```python
from build123d import *

# Parameters (mm, degrees)
SKETCH2_R           = 11.1125
BOSS_EXTRUDE1_DEPTH = 6.35


with BuildPart() as part:
    # Sketch2 → Boss-Extrude1 (new body)
    with BuildSketch(Plane.XY):
        with BuildLine():
            Line((0, 914.4), (-194.479849892, 914.4))
            ThreePointArc((-194.479849892, 914.4), (-204.91887294, 907.625287079), (-202.983200568, 895.332073104))
            ThreePointArc((-202.983200568, 895.332073104), (-164.535916973, 779.903104595), (-165.892020397, 658.247026365))
            Line((-165.892020397, 658.247026365), (-165.938886188, 658.129795086))
            ThreePointArc((-165.938886188, 658.129795086), (-174.522720833, 620.054602536), (-187.919807247, 583.395080165))
            ThreePointArc((-187.919807247, 583.395080165), (-210.62430537, 541.201744159), (-239.683438479, 503.105305725))
            ThreePointArc((-239.683438479, 503.105305725), (-421.799875663, 296.628923536), (-582.037423098, 72.747657042))
            ThreePointArc((-582.037423098, 72.747657042), (-620.339092238, 32.211350912), (-671.307126152, 9.573561873))
            ThreePointArc((-671.307126152, 9.573561873), (-674.990888604, 5.409489794), (-676.274252252, 0))
            ThreePointArc((-676.274252252, 0), (-674.990888604, -5.409489794), (-671.307126152, -9.573561873))
            ThreePointArc((-671.307126152, -9.573561873), (-620.339092238, -32.211350912), (-582.037423098, -72.747657042))
            ThreePointArc((-582.037423098, -72.747657042), (-421.799875663, -296.628923536), (-239.683438479, -503.105305725))
            ThreePointArc((-239.683438479, -503.105305725), (-191.627212465, -575.297388544), (-165.938886188, -658.129795086))
            Line((-165.938886188, -658.129795086), (-165.892020397, -658.247026365))
            ThreePointArc((-165.892020397, -658.247026365), (-164.535916973, -779.903104595), (-202.983200568, -895.332073104))
            ThreePointArc((-202.983200568, -895.332073104), (-204.91887294, -907.625287079), (-194.479849892, -914.4))
            Line((-194.479849892, -914.4), (0, -914.4))
            Line((0, -914.4), (194.479849892, -914.4))
            ThreePointArc((194.479849892, -914.4), (204.91887294, -907.625287079), (202.983200568, -895.332073104))
            ThreePointArc((202.983200568, -895.332073104), (164.535916973, -779.903104595), (165.892020397, -658.247026365))
            Line((165.892020397, -658.247026365), (165.938886188, -658.129795086))
            ThreePointArc((165.938886188, -658.129795086), (174.522720833, -620.054602536), (187.919807247, -583.395080165))
            ThreePointArc((187.919807247, -583.395080165), (210.62430537, -541.201744159), (239.683438479, -503.105305725))
            ThreePointArc((239.683438479, -503.105305725), (421.799875663, -296.628923536), (582.037423098, -72.747657043))
            ThreePointArc((582.037423098, -72.747657043), (620.339092238, -32.211350912), (671.307126152, -9.573561873))
            ThreePointArc((671.307126152, -9.573561873), (674.990888603, -5.409489794), (676.274252252, 0))
            ThreePointArc((676.274252252, 0), (674.990888604, 5.409489794), (671.307126152, 9.573561873))
            ThreePointArc((671.307126152, 9.573561873), (620.339092238, 32.211350912), (582.037423098, 72.747657042))
            ThreePointArc((582.037423098, 72.747657042), (421.799875663, 296.628923536), (239.683438479, 503.105305725))
            ThreePointArc((239.683438479, 503.105305725), (191.627212465, 575.297388544), (165.938886188, 658.129795086))
            Line((165.938886188, 658.129795086), (165.892020397, 658.247026365))
            ThreePointArc((165.892020397, 658.247026365), (164.535916973, 779.903104595), (202.983200568, 895.332073104))
            ThreePointArc((202.983200568, 895.332073104), (204.91887294, 907.625287079), (194.479849892, 914.4))
            Line((194.479849892, 914.4), (0, 914.4))
        make_face()
        with Locations((-58.541769794, -639.405335996)):
            Circle(SKETCH2_R, mode=Mode.SUBTRACT)
        with Locations((-58.541769794, -838.268909678)):
            Circle(SKETCH2_R, mode=Mode.SUBTRACT)
        with Locations((58.541769794, -838.268909678)):
            Circle(SKETCH2_R, mode=Mode.SUBTRACT)
        with Locations((58.541769794, -639.405335996)):
            Circle(SKETCH2_R, mode=Mode.SUBTRACT)
        with Locations((533.590599666, -57.767812484)):
            Circle(SKETCH2_R, mode=Mode.SUBTRACT)
        with Locations((330.356144827, -56.532187516)):
            Circle(SKETCH2_R, mode=Mode.SUBTRACT)
        with Locations((330.356144827, 56.532187516)):
            Circle(SKETCH2_R, mode=Mode.SUBTRACT)
        with Locations((533.590599666, 57.767812484)):
            Circle(SKETCH2_R, mode=Mode.SUBTRACT)
        with Locations((58.541769794, 838.268909678)):
            Circle(SKETCH2_R, mode=Mode.SUBTRACT)
        with Locations((-58.541769794, 838.268909678)):
            Circle(SKETCH2_R, mode=Mode.SUBTRACT)
        with Locations((-58.541769794, 639.405335996)):
            Circle(SKETCH2_R, mode=Mode.SUBTRACT)
        with Locations((58.541769794, 639.405335996)):
            Circle(SKETCH2_R, mode=Mode.SUBTRACT)
        with Locations((-330.356144827, -56.532187516)):
            Circle(SKETCH2_R, mode=Mode.SUBTRACT)
        with Locations((-330.356144827, 56.532187516)):
            Circle(SKETCH2_R, mode=Mode.SUBTRACT)
        with Locations((-533.590599666, 57.767812484)):
            Circle(SKETCH2_R, mode=Mode.SUBTRACT)
        with Locations((-533.590599666, -57.767812484)):
            Circle(SKETCH2_R, mode=Mode.SUBTRACT)
        with BuildLine():
            Line((294.116579618, 52.07611641), (294.116579618, -52.07611641))
            ThreePointArc((294.116579618, -52.07611641), (242.916605185, -291.544447454), (101.6983636, -491.604256507))
            ThreePointArc((101.6983636, -491.604256507), (89.07407881, -503.133976698), (76.131755899, -514.305516063))
            ThreePointArc((76.131755899, -514.305516063), (40.620898237, -536.014461284), (0, -545.083195538))
            ThreePointArc((0, -545.083195538), (-40.620898237, -536.014461284), (-76.131755899, -514.305516063))
            ThreePointArc((-76.131755899, -514.305516063), (-235.841357727, -307.108762007), (-294.116579618, -52.07611641))
            Line((-294.116579618, -52.07611641), (-294.116579618, 52.07611641))
            ThreePointArc((-294.116579618, 52.07611641), (-242.916605185, 291.544447454), (-101.6983636, 491.604256507))
            ThreePointArc((-101.6983636, 491.604256507), (-89.07407881, 503.133976698), (-76.131755899, 514.305516063))
            ThreePointArc((-76.131755899, 514.305516063), (-40.620898237, 536.014461284), (0, 545.083195538))
            ThreePointArc((0, 545.083195538), (40.620898237, 536.014461284), (76.131755899, 514.305516063))
            ThreePointArc((76.131755899, 514.305516063), (235.841357727, 307.108762007), (294.116579618, 52.07611641))
        make_face(mode=Mode.SUBTRACT)
    extrude(amount=BOSS_EXTRUDE1_DEPTH)


solid = part.part
```
The model under review builds one solid part; all positions refer to its coordinate system, in mm. A direction names the side the tool comes from. Give positions to 0.01 mm unless a question says otherwise; leave off trailing zeros. Write each loop counter-clockwise with the first axis right and the second up, starting at its lowest first coordinate (ties: lowest second). Pieces come first, ordered by that corner, then holes.
(1) Consider section D-D, the plane x = 461. Give the boundary of the cut face in (y, z).
(2) To check wall thickness, follow L1, parallel to Y at x = 340, z = 6.25; L2, parallel to Y at x = -67, z = 2.25; L3, parallel to Y at x = 64.5, z = 1.75. State the ranges of each line that lie inside material, in increasing order.
(3) Consider section A-A, the plane y = 251. Give the boundary of the cut face in (x, z), and give its area (3 significant figures).
(4) Tool access review of faces 1 (the cylindrical face through (620.98, 31.76, 3.13)), 2 (the cylindrical face through (234.26, 310.44, 3.13)): name each direction out of +Z, -Z, +X, -X, +Y, -Y from which nothing blocks a thin tool from reaching the whole face with its end or side.
(5) The part is to be moulded in two halves that separate along X. For faces 3 (the cylindrical face through (-192.15, -574.2, 3.13)), 4 (the cylindrical face through (-234.26, -310.44, 3.13)), 5 (the cylindrical face through (192.15, 574.2, 3.13)), say which applies: released by +X, released by -X, zero draft, split by the parting line, or undercut.
(6) Consider section B-B, the plane z = 5. Give the number of separate pieces and of enclosed holes in the cut face, and give its area (3 significant figures).
(7) Consider section C-C, the plane y = -473. Give the boundary of the cut face in (x, z), and give its area (3 significant figures).
(8) For P1, Ø18, axis at x = -533.59, y = 57.77, coming from the +Z side; P2, Ø3, axis at y = 445.5, z = 4.5, coming from the +X side; P3, Ø2, axis at x = -348, z = 5.5, coming from the +Y side; P4, Ø2, axis at y = 264.5, z = 1, coming from the -X side, all flat-tipped, find the tip position at first contact; note any pin that passes through.
Returned:
1. outline: (-246.14, 0) - (246.14, 0) - (246.14, 6.35) - (-246.14, 6.35) - close
2. L1: y = -394.63 to -62.05, -51.01 to 51.01, 62.05 to 394.63
2. L2: y = -914.4 to -845.48, -831.06 to -646.61, -632.2 to -521.5, 521.5 to 632.2, 646.61 to 831.06, 845.48 to 914.4
2. L3: y = -914.4 to -847.65, -828.89 to -648.79, -630.03 to -523.25, 523.25 to 630.03, 648.79 to 828.89, 847.65 to 914.4
3. outline: (-457.31, 0) - (-258.97, 0) - (-258.97, 6.35) - (-457.31, 6.35) - close; (258.97, 0) - (457.31, 0) - (457.31, 6.35) - (258.97, 6.35) - close
3. area: 2,520 mm2
4. face 1: +Z, -Z, +X, +Y
4. face 2: +Z, -Z
5. face 3: released by -X
5. face 4: undercut
5. face 5: released by +X
6. separate pieces: 1
6. enclosed holes: 17
6. area: 713,000 mm2
7. outline: (-268.64, 0) - (-120.66, 0) - (-120.66, 6.35) - (-268.64, 6.35) - close; (120.66, 0) - (268.64, 0) - (268.64, 6.35) - (120.66, 6.35) - close
7. area: 1,880 mm2
8. P1: passes through
8. P2: stops at x = 295.7
8. P3: stops at y = 386.6
8. P4: stops at x = -447.74
